Input: part model. Units: mm. Frame: model coordinates. Face numbers are marked on the shaded views. A direction names the side the tool comes from. Round coordinates to 2 decimals unless told otherwise and drop trailing zeros. Loops run counter-clockwise (first coordinate to the right, second up) from the corner with the lowest first, then second, coordinate; pieces in that order, holes last. Notation, with made-up numbers: (65.25, -29) - (112.25, -29) arc R12 cw to (112.25, -7) - close; hole circle Ø10 at (29.25, -36.5). An arc over 180 degrees is marked (long way). One line per question, with ' | ' between items. Start each with the question number.
from build123d import *

# Parameters (mm, degrees)
CYLINDER004_R     = 4.5
CYLINDER004_DEPTH = 12
CYLINDER_R        = 1.65
CYLINDER_DEPTH    = 8
BOX_W             = 8.74
BOX_H             = 16
BOX_DEPTH         = 7
FILLET012_R       = 0.6
FILLET013_R       = 3
CYLINDER006_R     = 4
CYLINDER006_DEPTH = 7
CYLINDER003_R     = 5.9
CYLINDER003_DEPTH = 10
CYLINDER002_R     = 7
CYLINDER002_DEPTH = 7
CHAMFER010_SIZE   = 0.4


with BuildPart() as cylinder004:
    # Cylinder004 → Cylinder004 (new body)
    with BuildSketch(Plane(origin=(6.5, 0, -3), x_dir=(1, 0, 0), z_dir=(0, 0, 1))):
        Circle(CYLINDER004_R)
    extrude(amount=CYLINDER004_DEPTH)


with BuildPart() as cylinder:
    # Cylinder → Cylinder (new body)
    with BuildSketch(Plane(origin=(0, 10, 0), x_dir=(1, 0, 0), z_dir=(0, 0, 1))):
        Circle(CYLINDER_R)
    extrude(amount=CYLINDER_DEPTH)


with BuildPart() as fillet013:
    # Box → Box (new body)
    with BuildSketch(Plane(origin=(-5.74, -3, 0), x_dir=(1, 0, 0), z_dir=(0, 0, 1))):
        with Locations((4.37, 8)):
            Rectangle(BOX_W, BOX_H)
    extrude(amount=BOX_DEPTH)

    # Fillet012
    fillet012_edges = [fillet013.edges().sort_by_distance(p)[0] for p in [
        (-5.74, -3, 3.5),
        (-5.74, 13, 3.5),
    ]]
    fillet(fillet012_edges, radius=FILLET012_R)

    # Fillet013
    fillet013_edges = [fillet013.edges().sort_by_distance(p)[0] for p in [
        (3, 13, 3.5),
    ]]
    fillet(fillet013_edges, radius=FILLET013_R)


with BuildPart() as cut002:
    # Cylinder006 → Cylinder006 (new body)
    with BuildSketch(Plane(origin=(0, 10, 0), x_dir=(1, 0, 0), z_dir=(0, 0, 1))):
        Circle(CYLINDER006_R)
    extrude(amount=CYLINDER006_DEPTH)

    # Fusion001: union Fillet013
    add(fillet013.part)

    # Cut002: cut Cylinder
    add(cylinder.part, mode=Mode.SUBTRACT)


with BuildPart() as cylinder003:
    # Cylinder003 → Cylinder003 (new body)
    with BuildSketch(Plane(origin=(6.5, 0, -3), x_dir=(1, 0, 0), z_dir=(0, 0, 1))):
        Circle(CYLINDER003_R)
    extrude(amount=CYLINDER003_DEPTH)


with BuildPart() as endstop_flag:
    # Cylinder002 → Cylinder002 (new body)
    with BuildSketch(Plane(origin=(6.5, 0, 0), x_dir=(1, 0, 0), z_dir=(0, 0, 1))):
        Circle(CYLINDER002_R)
    extrude(amount=CYLINDER002_DEPTH)

    # Fusion: union Cylinder003
    add(cylinder003.part)

    # Fusion002: union Cut002
    add(cut002.part)

    # Cut003: cut Cylinder004
    add(cylinder004.part, mode=Mode.SUBTRACT)

    # Chamfer010
    chamfer010_edges = [endstop_flag.edges().sort_by_distance(p)[0] for p in [
        (-2.482278, -3, 7),
        (-5.564264, -2.824264, 7),
        (-5.74, 5, 7),
        (-5.564264, 12.824264, 7),
        (-3.892876, 13, 7),
        (-1.65, 10, 0),
        (3, 6.708213, 7),
        (0.6, 0, -3),
        (8, 4.242641, 7),
        (2, 0, 7),
        (8, -4.242641, 7),
        (-1.65, 10, 7),
        (8.037549, -6.829051, 7),
        (10, 6.062178, 7),
        (3.741657, 8.585786, 7),
        (1.645751, 13.645751, 7),
    ]]
    chamfer(chamfer010_edges, length=CHAMFER010_SIZE)


solid = endstop_flag.part
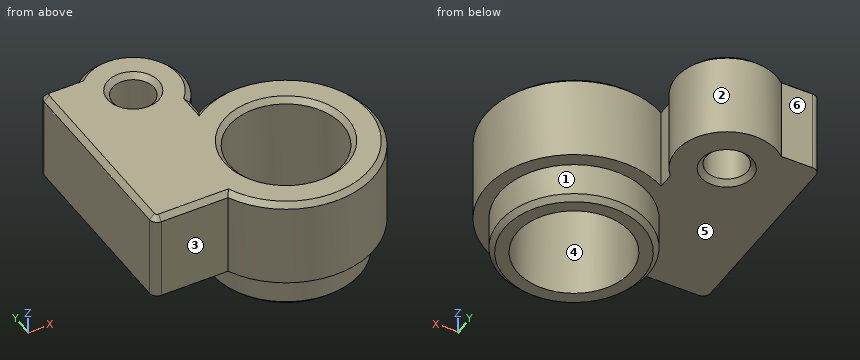
(1) Pull-direction query (Y, two-part tool) for the marked faces 4, 5 and 6; classes: released by +Y, released by -Y, zero draft, split by the parting line, or undercut.
(2) Section B-B, the plane z = 3.5. Output: boundary loops of the cut face in (x, y), plus the area to 3 significant figures.
(3) Section D-D, the plane y = 0. Output: boundary loops of the cut face in (x, z), plus the area to 3 significant figures.
(4) Line query: line 1 along Y through (x, z) = (0, 4); line 2 along Y through (x, z) = (6.5, 1); line 3 along X through (y, z) = (3.75, 5). Output: solid intervals per line, ascending. Write a range as from..to.
(5) Section C-C, the plane y = 10. Output: boundary loops of the cut face in (x, z), plus the area to 3 significant figures.
(6) Reachability of the marked faces 1, 2 and 3 from +Z, -Z, +X, -X, +Y, -Y: full face, straight path, thin tool, end or side. Return the list, or none.
(7) Pin query (flat end, axial travel): P1, Ø8, axis at x = 6.5, y = 0, coming from the +Z side; P2, Ø2, axis at x = -4, z = 2, coming from the +Y side; P3, Ø4, axis at x = 0, y = 10, coming from the -Z side; P4, Ø3, axis at y = 10, z = 2.5, coming from the +X side. Return the tip coordinate at first contact, or that it passes through.
(8) Section A-A, the plane x = 6.5. Output: boundary loops of the cut face in (y, z).
Derived:
1) face 4: undercut | face 5: zero draft | face 6: released by +Y
2) outline: (-5.74, -2.4) arc R0.6 ccw to (-5.14, -3) - (0.18, -3) arc R7 ccw (long way) to (3, 6.06) - (3, 7.35) arc R4 ccw to (-2.65, 13) - (-5.14, 13) arc R0.6 ccw to (-5.74, 12.4) - close; hole circle Ø3.3 at (0, 10); hole circle Ø9 at (6.5, 0) | area: 204 mm²
3) outline: (-5.74, 0) - (0.6, 0) - (0.6, -2.6) - (1, -3) - (2, -3) - (2, 6.6) - (1.6, 7) - (-5.34, 7) - (-5.74, 6.6) - close; (11, -3) - (12, -3) - (12.4, -2.6) - (12.4, 0) - (13.5, 0) - (13.5, 6.6) - (13.1, 7) - (11.4, 7) - (11, 6.6) - close | area: 79.6 mm²
4) line 1: y = -3..8.35, 11.65..14 | line 2: y = -7..-4.5, 4.5..7 | line 3: x = -5.74..4.01, 8.99..12.41
5) outline: (-5.74, 0) - (-2.05, 0) - (-1.65, 0.4) - (-1.65, 6.6) - (-2.05, 7) - (-5.34, 7) - (-5.74, 6.6) - close; (1.65, 0.4) - (2.05, 0) - (4, 0) - (4, 6.6) - (3.6, 7) - (2.05, 7) - (1.65, 6.6) - close | area: 44.6 mm²
6) face 1: -Z | face 2: +Z, -Z | face 3: +Z, -Z, -X, -Y
7) P1: passes through | P2: stops at y = 13 | P3: stops at z = 0.05 | P4: stops at x = 4
8) outline: (-7, 0) - (-5.9, 0) - (-5.9, -2.6) - (-5.5, -3) - (-4.5, -3) - (-4.5, 6.6) - (-4.9, 7) - (-6.6, 7) - (-7, 6.6) - close; (4.5, -3) - (5.5, -3) - (5.9, -2.6) - (5.9, 0) - (7, 0) - (7, 6.6) - (6.6, 7) - (4.9, 7) - (4.5, 6.6) - close
